Verification items for the finished model (mm, model axes). Coordinates: 2 decimals unless noted, no trailing zeros. Write each loop counter-clockwise with the first axis right and the second up, starting at its lowest first coordinate (ties: lowest second). Pieces come first, ordered by that corner, then holes. Notation, with made-up numbers: (81.5, 43) -> (124.5, 43) arc R26 ccw to (124.5, 60) -> close; hole circle Ø11 at (0.25, 56). An arc over 180 degrees is marked (long way). Answer in a Markdown table with one row per item.
```python
from build123d import *

# Parameters (mm, degrees)
BOSS_EXTRUDE1_DEPTH = 2
FILLET1_R           = 1
FILLET2_R           = 1
SKETCH2_R           = 2.5
CUT_EXTRUDE2_DEPTH  = 2


with BuildPart() as part:
    # Sketch1 → Boss-Extrude1 (new body)
    with BuildSketch(Plane.XY):
        with BuildLine():
            Line((-31.873882869, 46.769006648), (-31.873882869, 33.230993352))
            Line((-31.873882869, 33.230993352), (-73.208494435, 28.145662592))
            ThreePointArc((-73.208494435, 28.145662592), (-75.8185442, 40), (-73.208494435, 51.854337408))
            Line((-73.208494435, 51.854337408), (-31.873882869, 46.769006648))
        make_face()
    extrude(amount=BOSS_EXTRUDE1_DEPTH)

    # Fillet1
    fillet1_edges = [part.edges().sort_by_distance(p)[0] for p in [
        (-73.208494435, 51.854337408, 1),
        (-31.873882869, 46.769006648, 1),
        (-31.873882869, 33.230993352, 1),
        (-73.208494435, 28.145662592, 1),
    ]]
    fillet(fillet1_edges, radius=FILLET1_R)

    # Fillet2
    fillet2_edges = [part.edges().sort_by_distance(p)[0] for p in [
        (-52.613347795, 30.679450349, 2),
        (-75.8185442, 40, 2),
        (-31.873882869, 40, 2),
        (-52.613347795, 49.320549651, 2),
        (-32.124847572, 33.452974438, 2),
        (-32.124847572, 46.547025562, 2),
        (-73.094606247, 51.638989358, 2),
        (-73.094606247, 28.361010642, 2),
    ]]
    fillet(fillet2_edges, radius=FILLET2_R)

    # Sketch2 → Cut-Extrude2 (cut)
    with BuildSketch(Plane.XY.offset(2)):
        with Locations((-40, 40)):
            Circle(SKETCH2_R)
    extrude(amount=-CUT_EXTRUDE2_DEPTH, mode=Mode.SUBTRACT)


solid = part.part
```
1. Section check B-B, the plane z = 1.6. Record the boundary of the cut face in (x, y), plus the area to 3 significant figures.
Geometry says:
| item | result |
|---|---|
| outline | (-73.33, 28.91) arc R0.8 ccw to (-72.5, 28.43) -> (-32.78, 33.32) arc R0.8 ccw to (-32.07, 34.12) -> (-32.07, 45.88) arc R0.8 ccw to (-32.78, 46.68) -> (-72.5, 51.57) arc R0.8 ccw to (-73.33, 51.09) arc R28.03 ccw to start; hole circle Ø5 at (-40, 40) |
| area | 767 mm^2 |
2. Depth check by flat-ended pin: P1, Ø1, axis at x = -46.5, z = 1, coming from the +Y side. Enter the tip coordinate at first touch or a pass-through.
Geometry says:
| item | result |
|---|---|
| P1 | y = 48.63 |
3. Section check A-A, the plane y = 40. Record the boundary of the cut face in (x, z), plus the area to 3 significant figures.
Geometry says:
| item | result |
|---|---|
| outline | (-75.82, 0) -> (-42.5, 0) -> (-42.5, 2) -> (-74.82, 2) arc R1 ccw to (-75.82, 1) -> close; (-37.5, 0) -> (-31.87, 0) -> (-31.87, 1) arc R1 ccw to (-32.87, 2) -> (-37.5, 2) -> close |
| area | 77.5 mm^2 |
4. Mould release check, pull along X, two halves, no side actions. Record for faces 1 (the cylindrical face through (-52.37, 48.99, 1.71)), 2 (the cylindrical face through (-37.69, 39.04, 1.01)), 3 (the flat face through (-58, 40, 2)): released by +X, released by -X, zero draft, split by the parting line, or undercut.
Geometry says:
| item | result |
|---|---|
| face 1 | released by +X |
| face 2 | undercut |
| face 3 | zero draft |
5. Thickness scan on line 1 (Y direction, x = -38.5, z = 1.2); line 2 (Y direction, x = -40, z = 0.8); line 3 (Y direction, x = -45, z = 1.7). Record the ranges inside material, lowest first. Write a range as from..to.
Geometry says:
| item | result |
|---|---|
| line 1 | 32.44..38, 42..47.56 |
| line 2 | 32.23..37.5, 42.5..47.77 |
| line 3 | 31.9..48.1 |
